Autodesk Inventor part; units mm, degrees
ref_plane "YZ Plane" through (0, 0, 0) normal (1, 0, 0) x (0, 1, 0)
ref_plane "XZ Plane" through (0, 0, 0) normal (0, 1, 0) x (-1, 0, 0)
ref_plane "XY Plane" through (0, 0, 0) normal (0, 0, 1) x (1, 0, 0)
sketch "Sketch1" plane through (0, 0, 0) normal (0, 1, 0) x (-1, 0, 0)
  point P0 (0, 0)
sketch "Sketch2" plane through (0, 0, 0) normal (0, 1, 0) x (-1, 0, 0)
  line L0 (0, 0) -> (-122, 0)
  line L1 (-122, 0) -> (-122, -72)
  line L2 (-122, -72) -> (0, -72)
  line L3 (0, -72) -> (0, 0)
  dimension "d0" = 122
  dimension "d1" = 72
extrude "Extrusion1" add sketch "Sketch2" along normal blind 1
sketch "Sketch3" plane through (0, 1, 0) normal (0, 1, 0) x (1, 0, 0)
  line L0 (122, 72) -> (0, 72)
  line L1 (0, 72) -> (1, 72)
  line L2 (1, 72) -> (1, 71)
  line L3 (1, 71) -> (0, 71)
  line L4 (0, 71) -> (0, 72)
  line L5 (122, 0) -> (122, 72)
  line L6 (122, 0) -> (121, 0)
  line L7 (121, 0) -> (121, 1)
  line L8 (121, 1) -> (122, 1)
  line L9 (122, 1) -> (122, 0)
  line L10 (1, 71) -> (121, 71)
  line L11 (121, 71) -> (121, 1)
  line L12 (121, 1) -> (1, 1)
  line L13 (1, 1) -> (1, 71)
  line L14 (0, 71) -> (122, 71)
  line L15 (122, 71) -> (122, 0)
  line L16 (122, 0) -> (0, 0)
  line L17 (0, 0) -> (0, 71)
  dimension "d4" = 1
  dimension "d5" = 1
  dimension "d6" = 1
  dimension "d7" = 1
extrude "Extrusion2" add sketch "Sketch3" along normal blind 15 contours L5 L14 L10 L2 L0 | L2 L3 L4 L0 | L5 L8 L11 L14 | L13 L12 L7 L16 L17 L3 | L5 L6 L7 L8
sketch "Sketch5" plane through (0, 16, 0) normal (0, 1, 0) x (1, 0, 0)
  line L0 (0, 0) -> (122, 0)
  line L1 (0, 0) -> (0.5, 0)
  line L2 (0.5, 0) -> (0.5, 0.5)
  line L3 (0.5, 0.5) -> (0, 0.5)
  line L4 (0, 0.5) -> (0, 0)
  line L5 (122, 72) -> (121.5, 72)
  line L6 (121.5, 72) -> (121.5, 71.5)
  line L7 (121.5, 71.5) -> (122, 71.5)
  line L8 (122, 71.5) -> (122, 72)
  line L9 (121.5, 71.5) -> (0.5, 71.5)
  line L10 (0.5, 71.5) -> (0.5, 0.5)
  line L11 (0.5, 0.5) -> (121.5, 0.5)
  line L12 (121.5, 0.5) -> (121.5, 71.5)
  line L13 (121, 71) -> (121, 1)
  line L14 (1, 1) -> (1, 71)
  line L15 (121, 1) -> (1, 1)
  line L16 (1, 1) -> (1, 71)
  line L17 (1, 71) -> (121, 71)
  line L18 (121, 71) -> (121, 1)
  point P0 (121, 71)
  dimension "d10" = 0.5
  dimension "d11" = 0.5
  dimension "d12" = 0.5
  dimension "d13" = 0.5
extrude "Extrusion3" add sketch "Sketch5" along normal blind 5 contours L10 L9 L12 L11
properties part number "tapa"
Here's how the part is built. I have some questions about the finished solid (model axes, mm). A direction names the side the tool comes from. Coordinates: 2 decimals unless noted, no trailing zeros. Loops run counter-clockwise (first coordinate to the right, second up) from the corner with the lowest first, then second, coordinate; pieces in that order, holes last. Notation, with made-up numbers: (39.25, -33) - (78.25, -33) arc R8 cw to (78.25, -26) - close; hole circle Ø7 at (50, 31). An arc over 180 degrees is marked (long way). Return JSON: item names as keys, results as strings. Group by question number.
Item 1: If we section it at B-B on x = 105: Write out the boundary of the cut face in (y, z).
Item 2: We'd pull the mould along Z, two halves only. Please class faces 4 (the face through (121, 11, -36)), 5 (the face through (62, 11, -1)), 6 (the face through (62, 18, -71.5)), 7 (the face through (62, 0, -35)): +Z half, -Z half, draft (parallel to the pull), parting line (faces both ways), or undercut.
Item 3: I need wall thicknesses on line 1 (Z direction, x = 53, y = 4.25); line 2 (X direction, y = 14.75, z = -36.5); line 3 (Y direction, x = 102, z = -54). Which ranges of each line are inside material? Lowest first, please. Write a range as from..to.
Item 4: On a 3-axis mill with a long thin cutter (end or side, diameter ignored), from which of +Z, -Z, +X, -X, +Y, -Y can I reach the whole of each face in a straight line? I mean faces 1 (the face through (62, 1, -36)), 2 (the face through (60, 18, -0.5)), 3 (the face through (121.5, 18, -36)). Say none if no direction works.
Item 5: If we section it at A-A on y = 3.75: Write out the boundary of the cut face in (x, z).
Item 6: If we section it at C-C on z = -60.5: Write out the boundary of the cut face in (x, y), and give its area (3 significant figures).
Item 7: Will these pins go through, and if not, where does the flat tip stop? P1, Ø1.5, axis at x = 77, y = 19.5, coming from the +Z side; P2, Ø2.5, axis at y = 18.5, z = -39, coming from the -X side; P3, Ø5.5, axis at y = 19.5, z = -39, coming from the +X side.
Calculated:
{
 "1": {"outline": "(0, -72) - (16, -72) - (16, -71.5) - (21, -71.5) - (21, -71) - (1, -71) - (1, -1) - (21, -1) - (21, -0.5) - (16, -0.5) - (16, 0) - (0, 0) - close"},
 "2": {"face 4": "undercut", "face 5": "undercut", "face 6": "-Z half", "face 7": "draft"},
 "3": {"line 1": "z = -72..-71, -1..0", "line 2": "x = 0..1, 121..122", "line 3": "y = 0..1"},
 "4": {"face 1": "+Y", "face 2": "+Z, +X, -X, +Y", "face 3": "+Z, -Z, +X, +Y"},
 "5": {"outline": "(0, -72) - (122, -72) - (122, 0) - (0, 0) - close; hole (1, -71) - (121, -71) - (121, -1) - (1, -1) - close"},
 "6": {"outline": "(0, 0) - (122, 0) - (122, 16) - (121.5, 16) - (121.5, 21) - (121, 21) - (121, 1) - (1, 1) - (1, 21) - (0.5, 21) - (0.5, 16) - (0, 16) - close", "area": "157 mm^2"},
 "7": {"P1": "stops at z = -0.5", "P2": "stops at x = 0.5", "P3": "stops at x = 121.5"}
}
